```python
from build123d import *

# Parameters (mm, degrees)
F2_DEPTH = 25.4
F3_T     = -2.54


with BuildPart() as f2:
    # F1 (on face) → F2 (new body)
    with BuildSketch(Plane.XY):
        Polygon((-13.636127, 73.258446), (-70.261739, 24.819991), (-56.625612, -48.438456), (13.636127, -73.258446), (70.261739, -24.819991), (56.625612, 48.438456), align=None)
    extrude(amount=F2_DEPTH)

    # F3
    f3_openings = [f2.faces().sort_by_distance(p)[0] for p in [
        (0, 0, 25.4),
    ]]
    offset(amount=F3_T, openings=f3_openings)


solid = f2.part
```
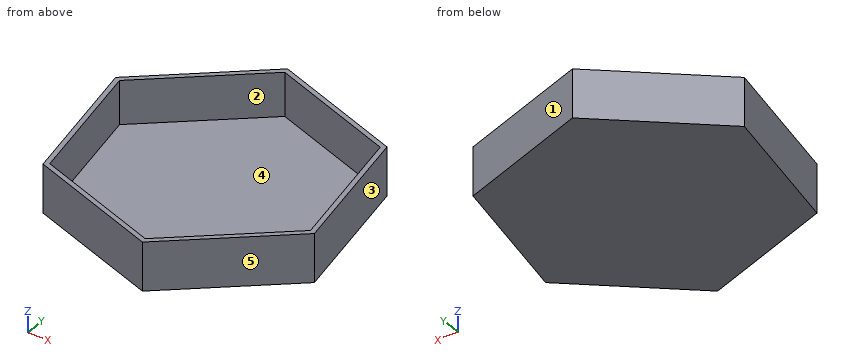
The model under review builds one solid part; all positions refer to its coordinate system, in mm. Face numbers are marked on the shaded views. A direction names the side the tool comes from. Round coordinates to 2 decimals unless told otherwise and drop trailing zeros. Order: outer loops, then holes, each group sorted by start corner. A loop starts at its lowest first (then second) coordinate and runs counter-clockwise, first axis right, second up. Notation, with made-up numbers: M 20,37.5 L 43,37.5 A22 cw 43,61.5 Z; hole C -28.5,-29 d4. An arc over 180 degrees is marked long. Use a Markdown table: item, result.
1) Insertion check: pin 1 (8 mm diameter, centred on x = -33.5, z = 13.5, fed in from +Y); pin 2 (8 mm diameter, centred on y = -11.5, z = 11.5, fed in from -X); pin 3 (3 mm diameter, centred on x = -4.5, z = 22.5, fed in from -Y). Each pin has a flat end and moves straight along its axis. Give the tip position at first contact, or say it passes through.
Report:
| item | result |
|---|---|
| pin 1 | y = 59.69 |
| pin 2 | x = -64.25 |
| pin 3 | y = -67.38 |
2) Draft analysis for pull direction Y (two halves, no side actions). For the marked faces 3, 4 and 5, state which applies: released by +Y, released by -Y, zero draft, split by the parting line, or undercut.
Report:
| item | result |
|---|---|
| face 3 | released by +Y |
| face 4 | undercut |
| face 5 | released by -Y |
3) Wall thickness on line 1 along Z through (x, y) = (6, 8.5); line 2 along Y through (x, z) = (54, 16); line 3 along X through (y, z) = (30, 23.5): over which ranges is each line inside the solid? List them lowest first. Write a range as [from, to].
Report:
| item | result |
|---|---|
| line 1 | [0, 2.54] |
| line 2 | [-38.73, -35.39], [46.67, 49.37] |
| line 3 | [-64.21, -60.3], [57.47, 60.06] |
4) Consider section C-C (y = 33). Write out the cut boundary in (x, z), then the cut area to 3 significant figures.
Report:
| item | result |
|---|---|
| outline | M -60.7,0 L 59.5,0 L 59.5,25.4 L 56.92,25.4 L 56.92,2.54 L -56.79,2.54 L -56.79,25.4 L -60.7,25.4 Z |
| area | 454 mm^2 |
5) Consider section B-B (x = -50). Write out the cut boundary in (y, z), then the cut area to 3 significant figures.
Report:
| item | result |
|---|---|
| outline | M -50.78,0 L 42.15,0 L 42.15,25.4 L 38.81,25.4 L 38.81,2.54 L -48.09,2.54 L -48.09,25.4 L -50.78,25.4 Z |
| area | 374 mm^2 |
6) Tool access review of the marked faces 1 and 2: name each direction out of +Z, -Z, +X, -X, +Y, -Y from which nothing blocks a thin tool from reaching the whole face with its end or side.
Report:
| item | result |
|---|---|
| face 1 | +Z, -Z, +X, +Y |
| face 2 | +Z |
7) Consider section A-A (z = 5.5). Write out the cut boundary in (x, y).
Report:
| item | result |
|---|---|
| outline | M -70.26,24.82 L -56.63,-48.44 L 13.64,-73.26 L 70.26,-24.82 L 56.63,48.44 L -13.64,73.26 Z; hole M -67.5,23.84 L -54.4,-46.53 L 13.1,-70.38 L 67.5,-23.84 L 54.4,46.53 L -13.1,70.38 Z |
